The figure shows three views and two pictorial views of one solid part (mm, origin at its lowest corner). Answer the questions. A direction names the side the tool comes from. Round coordinates to 2 decimals unless told otherwise and drop trailing zeros. Write each loop counter-clockwise with the first axis right and the second up, starting at its lowest first coordinate (ties: lowest second). Pieces come first, ordered by that corner, then holes. Notation, with made-up numbers: M 43.5,65 L 97.5,65 A11 cw 97.5,84 Z; hole C -2.5,3.25 d9. An arc over 180 degrees is marked long. One line per item, written item: value. Start each with the question number.
Q1. Given pin 1 Ø4 at (x, z) = (21.5, 4) entering from +Y; pin 2 Ø1.5 at (x, y) = (14, 3) entering from +Z; pin 3 Ø0.5 at (x, y) = (11.5, 1.5) entering from -Z; pin 4 Ø1.7 at (x, z) = (2, 2) entering from -Y, each flat-ended and moving along its own axis, determine where each tip first touches the part or whether it passes through.
Q2. Find section C-C (y = 0.65). Write down the section's boundary in (x, z).
Q3. Find section B-B (z = 14.5). Write down the section's boundary in (x, y), and give its area (3 significant figures).
Q4. Find section D-D (z = 7.5). Write down the section's boundary in (x, y), and give its area (3 significant figures).
Q5. Consider probe 1 along Z at (x, y) = (23, 0.2); probe 2 along X at (y, z) = (0.8, 14.5); probe 3 along Y at (x, z) = (13.25, 1.5). Determine where each line is inside the solid, lowest interval first.
Q6. Find section A-A (x = 23). Write down the section's boundary in (y, z), and give its area (3 significant figures).
Q7. A tool of negligible diameter and unlimited length cuts with its end or side. For the marked faces 1, 2, 3 and 4, from which of +Z, -Z, +X, -X, +Y, -Y can it reach the whole face along a straight path? Write none if from no direction.
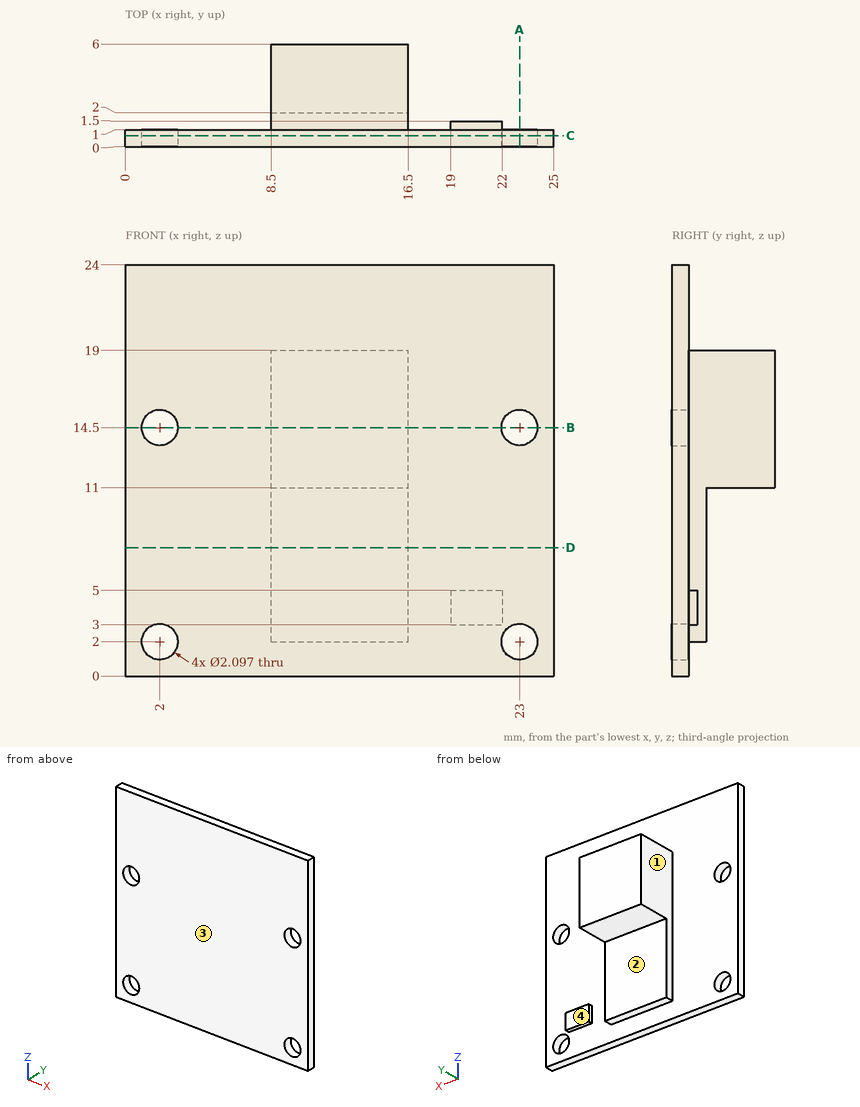
The answers:
1. pin 1: y = 1.5
1. pin 2: z = 19
1. pin 3: z = 2
1. pin 4: through
2. outline: M 0,0 L 25,0 L 25,24 L 0,24 Z; hole C 2,2 d2.1; hole C 2,14.5 d2.1; hole C 23,2 d2.1; hole C 23,14.5 d2.1
3. outline: M 0,0 L 0.95,0 L 0.95,1 L 0,1 Z; M 3.05,0 L 21.95,0 L 21.95,1 L 16.5,1 L 16.5,6 L 8.5,6 L 8.5,1 L 3.05,1 Z; M 24.05,0 L 25,0 L 25,1 L 24.05,1 Z
3. area: 60.8 mm2
4. outline: M 0,0 L 25,0 L 25,1 L 16.5,1 L 16.5,2 L 8.5,2 L 8.5,1 L 0,1 Z
4. area: 33.0 mm2
5. probe 1: 0 to 0.95, 3.05 to 13.45, 15.55 to 24
5. probe 2: 0 to 0.95, 3.05 to 21.95, 24.05 to 25
5. probe 3: 0 to 1
6. outline: M 0,0 L 1,0 L 1,0.95 L 0,0.95 Z; M 0,3.05 L 1,3.05 L 1,13.45 L 0,13.45 Z; M 0,15.55 L 1,15.55 L 1,24 L 0,24 Z
6. area: 19.8 mm2
7. face 1: +Z, -Z, -X, +Y
7. face 2: -Z, +X, -X, +Y
7. face 3: +Z, -Z, +X, -X, -Y
7. face 4: +Z, -Z, +X, +Y
